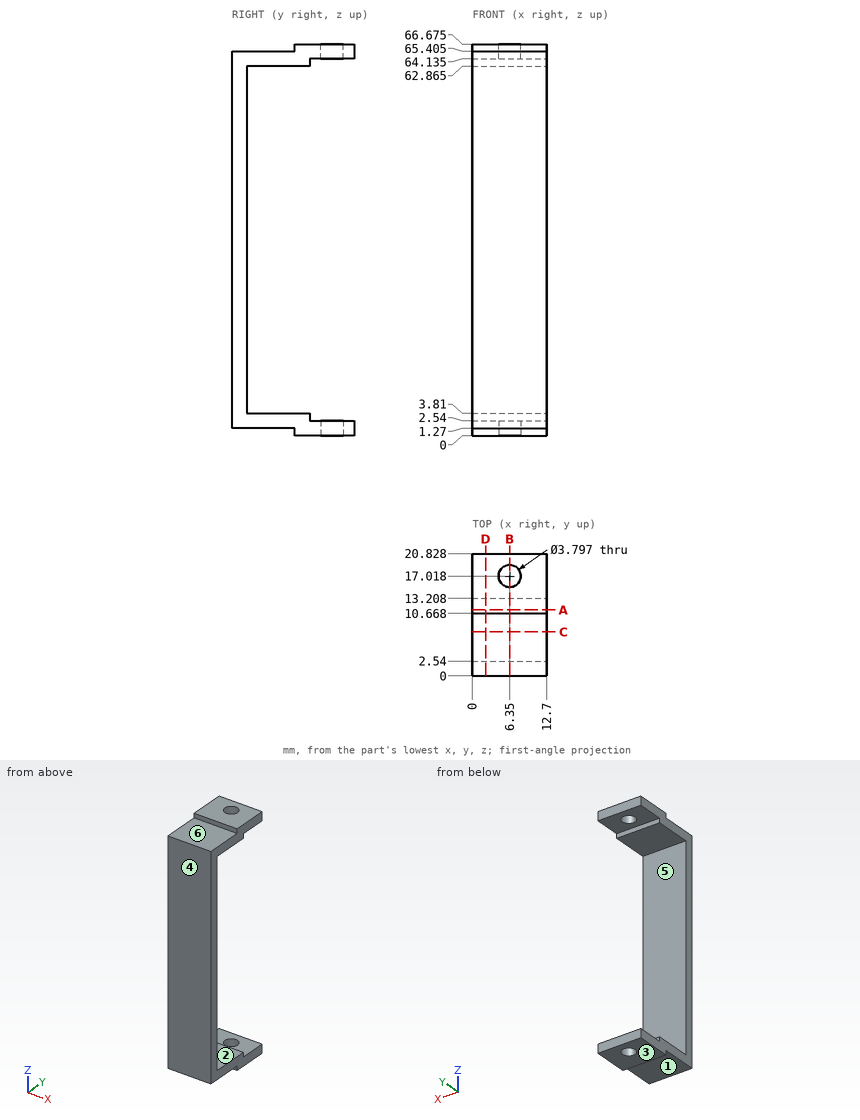
Design review of the part shown in the three views and the two pictorial views. Dimensions are in mm from the part's minimum x, y and z. A direction names the side the tool comes from. Give positions to 0.01 mm unless a question says otherwise; leave off trailing zeros. Write each loop counter-clockwise with the first axis right and the second up, starting at its lowest first coordinate (ties: lowest second). Pieces come first, ordered by that corner, then holes. Notation, with made-up numbers: M 54,79.25 L 98,79.25 A28 ccw 98,110.25 Z; hole C 32,66 d9. An arc over 180 degrees is marked long. Answer as CSV lines item,"result".
1. Draft analysis for pull direction Z (two halves, no side actions). For the marked faces 4, 5 and 6, state which applies: +Z half, -Z half, draft (parallel to the pull), parting line (faces both ways), or undercut.
Findings:
face 4,"draft"
face 5,"undercut"
face 6,"+Z half"
2. Wall thickness on line 1 (Z direction, x = 2.5, y = 4.5) (1 decimal); line 2 (Z direction, x = 1, y = 19) (1 decimal); line 3 (Y direction, x = 6.35, z = 0.95): over which ranges is each line inside the solid? List them lowest first.
Findings:
line 1,"z = 1.3 to 3.8, 62.9 to 65.4"
line 2,"z = 0 to 2.5, 64.1 to 66.7"
line 3,"y = 10.67 to 15.12, 18.92 to 20.83"
3. Consider section A-A, the plane y = 11.25. Write out the cut boundary in (x, z) (1 decimal).
Findings:
outline,"M 0,0 L 12.7,0 L 12.7,3.8 L 0,3.8 Z; M 0,62.9 L 12.7,62.9 L 12.7,66.7 L 0,66.7 Z"
4. Consider section C-C, the plane y = 7.5. Write out the cut boundary in (x, z) (1 decimal).
Findings:
outline,"M 0,1.3 L 12.7,1.3 L 12.7,3.8 L 0,3.8 Z; M 0,62.9 L 12.7,62.9 L 12.7,65.4 L 0,65.4 Z"
5. Consider section B-B, the plane x = 6.35. Write out the cut boundary in (y, z) (1 decimal), then the cut area to 3 significant figures.
Findings:
outline,"M 0,1.3 L 10.7,1.3 L 10.7,0 L 15.1,0 L 15.1,2.5 L 13.2,2.5 L 13.2,3.8 L 2.5,3.8 L 2.5,62.9 L 13.2,62.9 L 13.2,64.1 L 15.1,64.1 L 15.1,66.7 L 10.7,66.7 L 10.7,65.4 L 0,65.4 Z; M 18.9,0 L 20.8,0 L 20.8,2.5 L 18.9,2.5 Z; M 18.9,64.1 L 20.8,64.1 L 20.8,66.7 L 18.9,66.7 Z"
area,"243 mm2"
6. For pin 1 (1.5 mm diameter, centred on x = 9, y = 9.5, fed in from -Z); pin 2 (0.6 mm diameter, centred on x = 9, z = 66, fed in from -Y); pin 3 (3 mm diameter, centred on x = 7, z = 27.5, fed in from +Y), all flat-tipped, find the tip position at first contact; note any pin that passes through.
Findings:
pin 1,"stops at z = 1.27"
pin 2,"stops at y = 10.67"
pin 3,"stops at y = 2.54"
7. Consider section D-D, the plane x = 2.25. Write out the cut boundary in (y, z) (1 decimal), then the cut area to 3 significant figures.
Findings:
outline,"M 0,1.3 L 10.7,1.3 L 10.7,0 L 20.8,0 L 20.8,2.5 L 13.2,2.5 L 13.2,3.8 L 2.5,3.8 L 2.5,62.9 L 13.2,62.9 L 13.2,64.1 L 20.8,64.1 L 20.8,66.7 L 10.7,66.7 L 10.7,65.4 L 0,65.4 Z"
area,"262 mm2"
8. For the marked faces 1, 2 and 3, list the 3-axis set-ups (+Z, -Z, +X, -X, +Y, -Y) from which the entire face can be reached by the end or side of a thin tool; tool diameter is ignored.
Findings:
face 1,"-Z, +X, -X, -Y"
face 2,"+X, -X, +Y"
face 3,"-Z, +X, -X, +Y, -Y"
